Verification items for the finished model (mm, model axes). Face numbers are marked on the shaded views. Round coordinates to 2 decimals unless told otherwise and drop trailing zeros. Loops run counter-clockwise (first coordinate to the right, second up) from the corner with the lowest first, then second, coordinate; pieces in that order, holes last. Notation, with made-up numbers: (32, 54.25) -> (59, 54.25) arc R9 cw to (59, 59.25) -> close; hole circle Ø11 at (11, -32). An arc over 180 degrees is marked (long way). Use CSV: the item, a comma, the result in double quotes. Start each with the question number.
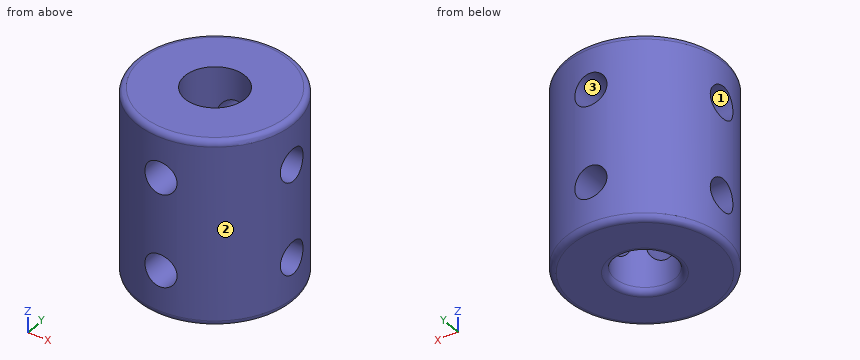
```python
from build123d import *

# Parameters (mm, degrees)
SKETCH1_R               = 6.825
SKETCH1_R_2             = 2.6
BOSS_EXTRUDE1_DEPTH     = 16
SKETCH3_R               = 1.4
CUT_EXTRUDE2_DEPTH      = 10
CIRPATTERN1_COUNT       = 4
FILLET1_R               = 0.5
MIRROR1_COPY_1_SKETCH_R = 1.4
MIRROR1_COPY_1_DEPTH    = 10
MIRROR1_COPY_2_SKETCH_R = 1.4
MIRROR1_COPY_2_DEPTH    = 10
MIRROR1_COPY_3_SKETCH_R = 1.4
MIRROR1_COPY_3_DEPTH    = 10


with BuildPart() as part:
    # Sketch1 → Boss-Extrude1 (new body)
    with BuildSketch(Plane.XY):
        Circle(SKETCH1_R)
        Circle(SKETCH1_R_2, mode=Mode.SUBTRACT)
    extrude(amount=BOSS_EXTRUDE1_DEPTH)

    # Sketch3 → Cut-Extrude2 (cut)
    with BuildSketch(Plane(origin=(0, 0, 0), x_dir=(1, 0, 0), z_dir=(0, 1, 0))):
        with Locations(Location((0, -12, 0), (0, 0, 270))):
            Circle(SKETCH3_R)
    cut_extrude2 = extrude(amount=-CUT_EXTRUDE2_DEPTH, mode=Mode.SUBTRACT)

    # CirPattern1: Cut-Extrude2 ×4 about axis
    cirpattern1_axis = Axis((0, 0, 16), (0, 0, -1))
    for i in range(1, CIRPATTERN1_COUNT):
        add(cut_extrude2.rotate(cirpattern1_axis, i * 360 / CIRPATTERN1_COUNT), mode=Mode.SUBTRACT)

    # Fillet1
    fillet1_edges = [part.edges().sort_by_distance(p)[0] for p in [
        (-6.825, 0, 0),
        (-6.825, 0, 16),
        (-2.6, 0, 0),
    ]]
    fillet(fillet1_edges, radius=FILLET1_R)

    # Mirror1: Cut-Extrude2 across plane
    add(cut_extrude2.mirror(Plane.XY.offset(8)), mode=Mode.SUBTRACT)

    # Mirror1 copy 1 sketch → Mirror1 copy 1 (cut)
    with BuildSketch(Plane(origin=(0, 0, 16), x_dir=(0, -1, 0), z_dir=(1, 0, 0))):
        with Locations((0, 12)):
            Circle(MIRROR1_COPY_1_SKETCH_R)
    extrude(amount=-MIRROR1_COPY_1_DEPTH, mode=Mode.SUBTRACT)

    # Mirror1 copy 2 sketch → Mirror1 copy 2 (cut)
    with BuildSketch(Plane(origin=(0, 0, 16), x_dir=(-1, 0, 0), z_dir=(0, -1, 0))):
        with Locations((0, 12)):
            Circle(MIRROR1_COPY_2_SKETCH_R)
    extrude(amount=-MIRROR1_COPY_2_DEPTH, mode=Mode.SUBTRACT)

    # Mirror1 copy 3 sketch → Mirror1 copy 3 (cut)
    with BuildSketch(Plane(origin=(0, 0, 16), x_dir=(0, 1, 0), z_dir=(-1, 0, 0))):
        with Locations((0, 12)):
            Circle(MIRROR1_COPY_3_SKETCH_R)
    extrude(amount=-MIRROR1_COPY_3_DEPTH, mode=Mode.SUBTRACT)


solid = part.part
```
Q1. Cross-section at C-C (z = 12.5). Record the boundary of the cut face in (x, y) (3 decimals).
Q2. Thickness scan on L1, parallel to Z at x = 0, y = 4; L2, parallel to X at y = 0, z = 10.5 (3 decimals); L3, parallel to Z at x = -4.25, y = 0.5. Record the ranges inside material, lowest first. Write a range as from..to.
Q3. Cross-section at D-D (z = 7.5). Record the boundary of the cut face in (x, y) (3 decimals), and give its area (3 significant figures).
Q4. Cross-section at A-A (x = 0). State how many separate pieces and enclosed holes the cut face has, and give its area (3 significant figures).
Q5. Depth check by flat-ended pin: pin 1 Ø1.5 at (x, z) = (-2, 4.5) entering from +Y. Enter the tip coordinate at first touch or a pass-through.
Q6. Release check for a two-part mould opening along X. For the marked faces 1, 2 and 3 record: +X half, -X half, draft (parallel to the pull), parting line (faces both ways), or undercut.
Answer list:
1,outline,"(-6.699, -1.308) arc R6.825 ccw to (-1.308, -6.699) -> (-1.308, -2.247) arc R2.6 cw to (-2.247, -1.308) -> close; (-6.699, 1.308) -> (-2.247, 1.308) arc R2.6 cw to (-1.308, 2.247) -> (-1.308, 6.699) arc R6.825 ccw to start; (1.308, -6.699) arc R6.825 ccw to (6.699, -1.308) -> (2.247, -1.308) arc R2.6 cw to (1.308, -2.247) -> close; (1.308, 2.247) arc R2.6 cw to (2.247, 1.308) -> (6.699, 1.308) arc R6.825 ccw to (1.308, 6.699) -> close"
2,L1,"z = 0..2.6, 5.4..10.6, 13.4..16"
2,L2,"x = -6.825..-2.6, 2.6..6.825"
2,L3,"z = 0..2.69, 5.31..10.69, 13.31..16"
3,outline,"circle Ø13.65 at (0, 0); hole circle Ø5.2 at (0, 0)"
3,area,"125 mm2"
4,separate pieces,"6"
4,enclosed holes,"0"
4,area,"87.6 mm2"
5,pin 1,"stops at y = 6.71"
6,face 1,"draft"
6,face 2,"parting line"
6,face 3,"undercut"
